Geometry check sheet. Reference: the model listing, model coordinates, mm. A direction names the side the tool comes from. Coordinates: 2 decimals unless noted, no trailing zeros. Order: outer loops, then holes, each group sorted by start corner. A loop starts at its lowest first (then second) coordinate and runs counter-clockwise, first axis right, second up. Notation, with made-up numbers: (41.25, -25.5) -> (74.25, -25.5) arc R29 ccw to (74.25, 4.5) -> close; hole circle Ø7 at (-7, -17). An arc over 180 degrees is marked (long way). Answer as CSV lines item,"result". Start each with the question number.
Autodesk Inventor part; units mm, degrees
ref_plane "YZ Plane" through (0, 0, 0) normal (1, 0, 0) x (0, 1, 0)
ref_plane "XZ Plane" through (0, 0, 0) normal (0, 1, 0) x (-1, 0, 0)
ref_plane "XY Plane" through (0, 0, 0) normal (0, 0, 1) x (1, 0, 0)
sketch "Sketch1" plane through (0, 0, 0) normal (0, 1, 0) x (-1, 0, 0)
  circle A0 centre (0, 0) radius 60
  dimension "d0" = 120
extrude "Extrusion1" add sketch "Sketch1" along normal blind 11
sketch "Sketch3" plane through (0, 11, 0) normal (0, 1, 0) x (1, 0, 0)
  circle A0 centre (0, 0) radius 40
  dimension "d6" = 80
extrude "Extrusion3" cut sketch "Sketch3" against normal through all
sketch "Sketch2" plane through (0, 0, 0) normal (0, -1, 0) x (1, 0, 0)
  circle A0 centre (0, 0) radius 50
  dimension "d3" = 100
extrude "Extrusion2" cut sketch "Sketch2" against normal blind 8
sketch "Sketch4" plane through (0, 11, 0) normal (0, 1, 0) x (1, 0, 0)
  circle A0 centre (0, 0) radius 55
  circle A1 centre (0, 55) radius 1.5
  circle A2 centre (-55, 0) radius 1.5
  circle A3 centre (0, -55) radius 1.5
  circle A4 centre (55, 0) radius 1.5
  dimension "d9" = 110
  dimension "d10" = 3
  dimension "d13" = 360
hole "Hole1" at (0, 11, -55) at (-55, 11, 0) at (0, 11, 55) at (55, 11, 0) direction (0, -1, 0) diameter 3 end through all countersink diameter 6 countersink angle 90
thread "Thread1"
thread "Thread2"
thread "Thread3"
thread "Thread4"
properties part number "sensor2_lock" material "Aluminum 6061"
Q1. Release check for a two-part mould opening along Z. For faces 1 (the cylindrical face through (59.94, 5.42, -2.64)), 2 (the cylindrical face through (-0.45, 4.68, 56.43)), 3 (the flat face through (-13, 0, -49)) record: released by +Z, released by -Z, zero draft, split by the parting line, or undercut.
Q2. Sectioned sample at D-D, the plane x = 24. Record the cut outline in (y, z), then the cut area to 3 significant figures.
Q3. Sectioned sample at C-C, the plane y = 6.25. Record the cut outline in (x, z).
Q4. Access from +Z, -Z, +X, -X, +Y, -Y to the whole of each face (thin tool, end or side, straight path). Record for faces 4 (the conical face through (0, 10, 57)), 5 (the cylindrical face through (47.69, 3.94, 15.02)).
Q5. Sectioned sample at B-B, the plane z = 36. Record the cut outline in (x, y).
Q6. Sectioned sample at A-A, the plane x = 0. Record the cut outline in (y, z), then the cut area to 4 significant figures.
Q7. Thickness scan on L1, parallel to Z at x = 0, y = 5; L2, parallel to Z at x = 0, y = 8.8; L3, parallel to Y at x = 32, z = -25. Record the ranges inside material, lowest first.
Q8. Go/stop test with flat-tipped pins: pin 1 Ø12 at (x, z) = (-14.5, -36.5) entering from -Y; pin 2 Ø4 at (x, z) = (55, 0) entering from +Y; pin 3 Ø1.5 at (y, z) = (9, -32) entering from -X; pin 4 Ø8 at (x, z) = (11.5, 37) entering from +Y. Record where each tip stops, or that it passes through.
Geometry results:
1,face 1,"split by the parting line"
1,face 2,"undercut"
1,face 3,"zero draft"
2,outline,"(0, -54.99) -> (11, -54.99) -> (11, -32) -> (8, -32) -> (8, -43.86) -> (0, -43.86) -> close; (0, 43.86) -> (8, 43.86) -> (8, 32) -> (11, 32) -> (11, 54.99) -> (0, 54.99) -> close"
2,area,"316 mm^2"
3,outline,"circle Ø120 at (0, 0); hole circle Ø3 at (-55, 0); hole circle Ø100 at (0, 0); hole circle Ø3 at (0, -55); hole circle Ø3 at (0, 55); hole circle Ø3 at (55, 0)"
4,face 4,"+Y"
4,face 5,"-Y"
5,outline,"(-48, 0) -> (-34.7, 0) -> (-34.7, 8) -> (-17.44, 8) -> (-17.44, 11) -> (-48, 11) -> close; (17.44, 8) -> (34.7, 8) -> (34.7, 0) -> (48, 0) -> (48, 11) -> (17.44, 11) -> close"
6,outline,"(0, -60) -> (11, -60) -> (11, -58) -> (9.5, -56.5) -> (0, -56.5) -> close; (0, -53.5) -> (9.5, -53.5) -> (11, -52) -> (11, -40) -> (8, -40) -> (8, -50) -> (0, -50) -> close; (0, 50) -> (8, 50) -> (8, 40) -> (11, 40) -> (11, 52) -> (9.5, 53.5) -> (0, 53.5) -> close; (0, 56.5) -> (9.5, 56.5) -> (11, 58) -> (11, 60) -> (0, 60) -> close"
6,area,"209.5 mm^2"
7,L1,"z = -60 to -56.5, -53.5 to -50, 50 to 53.5, 56.5 to 60"
7,L2,"z = -60 to -56.5, -53.5 to -40, 40 to 53.5, 56.5 to 60"
7,L3,"y = 8 to 11"
8,pin 1,"stops at y = 8"
8,pin 2,"stops at y = 10"
8,pin 3,"stops at x = -51.22"
8,pin 4,"stops at y = 11"
